For this review, use the dimensioned drawing (mm, ordinates from the lowest corner) and the shaded views. A direction names the side the tool comes from. Coordinates: 2 decimals unless noted, no trailing zeros. Loops run counter-clockwise (first coordinate to the right, second up) from the corner with the lowest first, then second, coordinate; pieces in that order, holes last. Notation, with made-up numbers: M 61,84.25 L 85,84.25 A8 cw 85,94.25 Z; hole C -8,10.5 d7. An arc over 180 degrees is marked long. Write item = value, one per line.
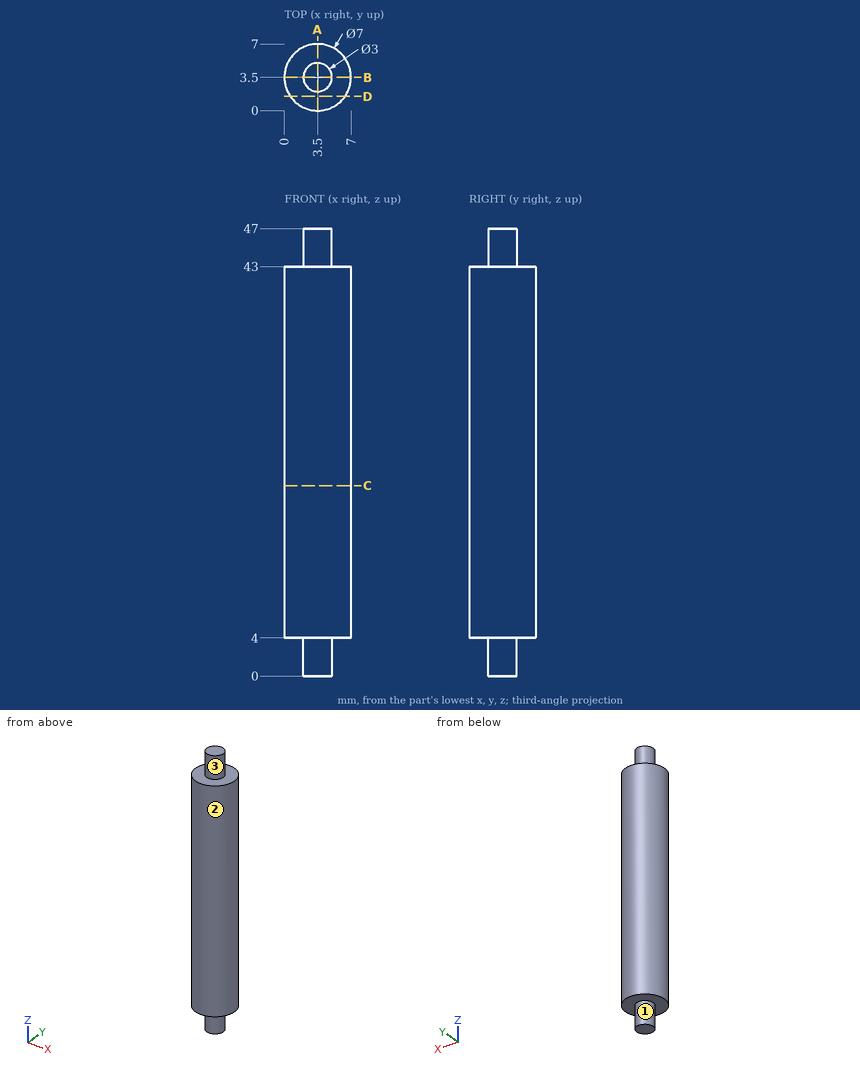
Q1. Machinability: for the marked faces 1, 2 and 3, which of the approach directions +Z, -Z, +X, -X, +Y, -Y give a long, thin tool a straight path to every point of the face, cutting with its end or side? Answer none if there is none.
Solved:
face_1 = -Z
face_2 = +Z, -Z
face_3 = +Z
Q2. Add section A-A (x = 3.5). Write out the cut boundary in (y, z), and give its area (3 significant figures).
Solved:
outline = M 0,4 L 2,4 L 2,0 L 5,0 L 5,4 L 7,4 L 7,43 L 5,43 L 5,47 L 2,47 L 2,43 L 0,43 Z
area = 297 mm²
Q3. For pin 1 Ø1.5 at (y, z) = (2, 23.5) entering from +X; pin 2 Ø3 at (x, z) = (1.5, 35) entering from +Y; pin 3 Ø1.5 at (y, z) = (2.5, 19) entering from -X, all flat-tipped, find the tip position at first contact; note any pin that passes through.
Solved:
pin_1 = 6.92
pin_2 = 6.96
pin_3 = 0.01
Q4. Add section D-D (y = 1.5). Write out the cut boundary in (x, z).
Solved:
outline = M 0.63,4 L 6.37,4 L 6.37,43 L 0.63,43 Z
Q5. For line 1 along Z through (x, y) = (5.25, 3.5); line 2 along X through (y, z) = (3.75, 7.5); line 3 along X through (y, z) = (0.5, 14.5), list the stretches that pass through material, from the lowest coordinate up.
Solved:
line_1 = 4 to 43
line_2 = 0.01 to 6.99
line_3 = 1.7 to 5.3
Q6. Add section C-C (z = 20). Write out the cut boundary in (x, y), and give its area (3 significant figures).
Solved:
outline = C 3.5,3.5 d7
area = 38.5 mm²
